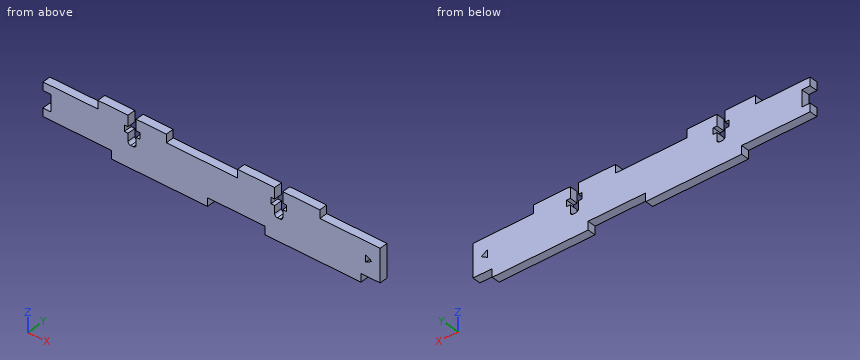
from build123d import *

# Parameters (mm, degrees)
SKETCH1_W                = 123
SKETCH1_H                = 12
BOSS_EXTRUDE1_DEPTH      = 1.5
SKETCH2_W                = 30
SKETCH2_H                = 3
BOSS_EXTRUDE2_DEPTH      = 1.5
SKETCH12_W               = 25
SKETCH12_H               = 3
BOSS_EXTRUDE3_DEPTH      = 1.5
CUT_EXTRUDE8_DEPTH       = 2.5
CUT_EXTRUDE8_DEPTH_BACK  = 2.5
SKETCH13_W               = 35
SKETCH13_H               = 3
BOSS_EXTRUDE4_DEPTH      = 1.5
CUT_EXTRUDE10_DEPTH      = 2.5
CUT_EXTRUDE10_DEPTH_BACK = 2.5
SKETCH16_W               = 3
SKETCH16_H               = 6
CUT_EXTRUDE11_DEPTH      = 2.5
CUT_EXTRUDE11_DEPTH_BACK = 2.5


with BuildPart() as part:
    # Sketch1 → Boss-Extrude1 (new body, symmetric)
    with BuildSketch(Plane(origin=(0, 0, 0), x_dir=(1, 0, 0), z_dir=(0, 1, 0))):
        Rectangle(SKETCH1_W, SKETCH1_H)
    extrude(amount=BOSS_EXTRUDE1_DEPTH, both=True)

    # Sketch2 → Boss-Extrude2 (add, symmetric)
    with BuildSketch(Plane(origin=(0, 0, 0), x_dir=(1, 0, 0), z_dir=(0, 1, 0))):
        with Locations((24.5, -7.5)):
            Rectangle(SKETCH2_W, SKETCH2_H)
    extrude(amount=BOSS_EXTRUDE2_DEPTH, both=True)

    # Sketch12 → Boss-Extrude3 (add, symmetric)
    with BuildSketch(Plane(origin=(0, 0, 0), x_dir=(1, 0, 0), z_dir=(0, 1, 0))):
        with Locations((-29, -7.5)):
            Rectangle(SKETCH12_W, SKETCH12_H)
    extrude(amount=BOSS_EXTRUDE3_DEPTH, both=True)

    # Sketch11 → Cut-Extrude8 (cut, two sides)
    with BuildSketch(Plane(origin=(0, 0, 0), x_dir=(1, 0, 0), z_dir=(0, 1, 0))) as cut_extrude8_sk:
        with BuildLine():
            Line((-30.5, -9), (-27.5, -9))
            Line((-27.5, -9), (-27.5, -5))
            Line((-27.5, -5), (-26.15, -5))
            Line((-26.15, -5), (-26.15, -2.73))
            Line((-26.15, -2.73), (-27.5, -2.73))
            Line((-27.5, -2.73), (-27.5, 0))
            ThreePointArc((-27.5, 0), (-27.792893219, 0.707106781), (-28.5, 1))
            Line((-28.5, 1), (-29.5, 1))
            ThreePointArc((-29.5, 1), (-30.207106781, 0.707106781), (-30.5, 0))
            Line((-30.5, 0), (-30.5, -2.73))
            Line((-30.5, -2.73), (-31.85, -2.73))
            Line((-31.85, -2.73), (-31.85, -5))
            Line((-31.85, -5), (-30.5, -5))
            Line((-30.5, -5), (-30.5, -9))
        make_face()
        with BuildLine():
            Line((23, -9), (26, -9))
            Line((26, -9), (26, -5))
            Line((26, -5), (27.35, -5))
            Line((27.35, -5), (27.35, -2.73))
            Line((27.35, -2.73), (26, -2.73))
            Line((26, -2.73), (26, 0))
            ThreePointArc((26, 0), (25.707106781, 0.707106781), (25, 1))
            Line((25, 1), (24, 1))
            ThreePointArc((24, 1), (23.292893219, 0.707106781), (23, 0))
            Line((23, 0), (23, -2.73))
            Line((23, -2.73), (21.65, -2.73))
            Line((21.65, -2.73), (21.65, -5))
            Line((21.65, -5), (23, -5))
            Line((23, -5), (23, -9))
        make_face()
    extrude(amount=CUT_EXTRUDE8_DEPTH, mode=Mode.SUBTRACT)
    extrude(cut_extrude8_sk.sketch, amount=-CUT_EXTRUDE8_DEPTH_BACK, mode=Mode.SUBTRACT)

    # Sketch13 → Boss-Extrude4 (add, symmetric)
    with BuildSketch(Plane(origin=(0, 0, 0), x_dir=(1, 0, 0), z_dir=(0, 1, 0))):
        with Locations((-19, 7.5)):
            Rectangle(SKETCH13_W, SKETCH13_H)
        with Locations((37, 7.5)):
            Rectangle(SKETCH13_W, SKETCH13_H)
    extrude(amount=BOSS_EXTRUDE4_DEPTH, both=True)

    # Sketch15 → Cut-Extrude10 (cut, two sides)
    with BuildSketch(Plane(origin=(0, 0, 0), x_dir=(1, 0, 0), z_dir=(0, 1, 0))) as cut_extrude10_sk:
        Polygon((56.25, -1.299038106), (58.5, 0), (56.25, 1.299038106), align=None)
    extrude(amount=CUT_EXTRUDE10_DEPTH, mode=Mode.SUBTRACT)
    extrude(cut_extrude10_sk.sketch, amount=-CUT_EXTRUDE10_DEPTH_BACK, mode=Mode.SUBTRACT)

    # Sketch16 → Cut-Extrude11 (cut, two sides)
    with BuildSketch(Plane(origin=(0, 0, 0), x_dir=(1, 0, 0), z_dir=(0, 1, 0))) as cut_extrude11_sk:
        with Locations((-60, 0)):
            Rectangle(SKETCH16_W, SKETCH16_H)
    extrude(amount=CUT_EXTRUDE11_DEPTH, mode=Mode.SUBTRACT)
    extrude(cut_extrude11_sk.sketch, amount=-CUT_EXTRUDE11_DEPTH_BACK, mode=Mode.SUBTRACT)


solid = part.part
Read the model definition and answer for the solid it produces. Units are mm, in the model's axes. Coordinates: 2 decimals unless noted, no trailing zeros. Loops run counter-clockwise (first coordinate to the right, second up) from the corner with the lowest first, then second, coordinate; pieces in that order, holes last.
Q1. The part is cut by section B-B on z = -7.5. Write down the section's boundary in (x, y), and give its area (3 significant figures).
Q2. Consider probe 1 along X at (y, z) = (0.9, 1.75); probe 2 along X at (y, z) = (-0.35, 7.5); probe 3 along X at (y, z) = (-0.3, 4.25). Determine where each line is inside the solid, lowest interval first.
Q3. The part is cut by section A-A on z = 7.25. Write down the section's boundary in (x, y), and give its area (3 significant figures).
Q4. The part is cut by section D-D on x = -13.5. Write down the section's boundary in (y, z), and give its area (3 significant figures).
Q5. The part is cut by section C-C on x = 3.5. Write down the section's boundary in (y, z).
Q6. Each of these flat-tipped pins is pushed along its axis until it touches: pin 1 Ø1.5 at (y, z) = (0.5, 8) entering from -X; pin 2 Ø0.5 at (x, y) = (-29, 0.5) entering from +Z; pin 3 Ø1.5 at (y, z) = (-0.5, -0.5) entering from -X. Where does it stop, or does it pass through?
Results below:
1. outline: (-36.5, -1.5) - (-1.5, -1.5) - (-1.5, 1.5) - (-36.5, 1.5) - close; (19.5, -1.5) - (54.5, -1.5) - (54.5, 1.5) - (19.5, 1.5) - close
1. area: 210 mm2
2. probe 1: x = -58.5 to -30.5, -27.5 to 23, 26 to 61.5
2. probe 2: x = -41.5 to -30.5, -27.5 to -16.5, 9.5 to 23, 26 to 39.5
2. probe 3: x = -61.5 to -31.85, -26.15 to 21.65, 27.35 to 61.5
3. outline: (-41.5, -1.5) - (-30.5, -1.5) - (-30.5, 1.5) - (-41.5, 1.5) - close; (-27.5, -1.5) - (-16.5, -1.5) - (-16.5, 1.5) - (-27.5, 1.5) - close; (9.5, -1.5) - (23, -1.5) - (23, 1.5) - (9.5, 1.5) - close; (26, -1.5) - (39.5, -1.5) - (39.5, 1.5) - (26, 1.5) - close
3. area: 147 mm2
4. outline: (-1.5, -9) - (1.5, -9) - (1.5, 6) - (-1.5, 6) - close
4. area: 45.0 mm2
5. outline: (-1.5, -6) - (1.5, -6) - (1.5, 6) - (-1.5, 6) - close
6. pin 1: stops at x = -41.5
6. pin 2: stops at z = -1
6. pin 3: stops at x = -58.5
